Could you check a few things on this model? Use its own coordinates, in mm. A direction names the side the tool comes from. Give positions to 0.01 mm unless a question says otherwise; leave off trailing zeros. Loops run counter-clockwise (first coordinate to the right, second up) from the corner with the lowest first, then second, coordinate; pieces in that order, holes last. Notation, with made-up numbers: M 30,57.25 L 56,57.25 A34 ccw 56,90.25 Z; hole C 44.25,18 d6. An arc over 180 degrees is marked long. Use CSV: the item, a comma, the result in double quotes.
```python
from build123d import *

# Parameters (mm, degrees)
ESQUISSE1_R             = 12.5
BOSS_EXTRU_1_DEPTH      = 17
ESQUISSE2_R             = 12.5
BOSS_EXTRU_2_DEPTH      = 7
BOSS_EXTRU_2_TAPER      = 35
ESQUISSE3_R             = 1.5
ENL_V_MAT_EXTRU_1_DEPTH = 10
CONG_1_SIZE             = 0.5
ESQUISSE4_R             = 3.5
BOSS_EXTRU_3_DEPTH      = 2
ESQUISSE5_R             = 1.15
BOSS_EXTRU_4_DEPTH      = 13


with BuildPart() as part:
    # Esquisse1 → Boss.-Extru.1 (new body)
    with BuildSketch(Plane.XY):
        Circle(ESQUISSE1_R)
    extrude(amount=BOSS_EXTRU_1_DEPTH)

    # Esquisse2 → Boss.-Extru.2 (add)
    with BuildSketch(Plane.XY.offset(17)):
        Circle(ESQUISSE2_R)
    extrude(amount=BOSS_EXTRU_2_DEPTH, taper=BOSS_EXTRU_2_TAPER)

    # Esquisse3 → Enlèv. mat.-Extru.1 (cut)
    with BuildSketch(Plane(origin=(0, 0, 0), x_dir=(-1, 0, 0), z_dir=(0, 0, -1))):
        with Locations((-8, 0)):
            Circle(ESQUISSE3_R)
        with Locations((8, 0)):
            Circle(ESQUISSE3_R)
    extrude(amount=-ENL_V_MAT_EXTRU_1_DEPTH, mode=Mode.SUBTRACT)

    # Congé1
    # a fillet whose section is not a circle: 0.5 mm, written as the material it takes off along each edge
    with BuildSketch(Plane(origin=(-8, 0, 0), x_dir=(-1, 0, 0), z_dir=(0, -1, 0))) as cong_1_piece_1:
        with BuildLine():
            Bezier((1.5 + CONG_1_SIZE, 0), (1.5, 0), (1.5, -CONG_1_SIZE), weights=[1, 0.035355339, 1])
            Line((1.5, -CONG_1_SIZE), (1.5, 0))
            Line((1.5, 0), (1.5 + CONG_1_SIZE, 0))
        make_face()
    revolve(axis=Axis((-8, 0, 0), (0, 0, -1)), mode=Mode.SUBTRACT)
    with BuildSketch(Plane(origin=(8, 0, 0), x_dir=(-1, 0, 0), z_dir=(0, -1, 0))) as cong_1_piece_2:
        with BuildLine():
            Bezier((1.5 + CONG_1_SIZE, 0), (1.5, 0), (1.5, -CONG_1_SIZE), weights=[1, 0.035355339, 1])
            Line((1.5, -CONG_1_SIZE), (1.5, 0))
            Line((1.5, 0), (1.5 + CONG_1_SIZE, 0))
        make_face()
    revolve(axis=Axis((8, 0, 0), (0, 0, -1)), mode=Mode.SUBTRACT)

    # Esquisse4 → Boss.-Extru.3 (add)
    with BuildSketch(Plane(origin=(0, 0, 0), x_dir=(-1, 0, 0), z_dir=(0, 0, -1))):
        with Locations(Location((0, 0, 0), (0, 0, 180))):
            Circle(ESQUISSE4_R)
    extrude(amount=BOSS_EXTRU_3_DEPTH)

    # Esquisse5 → Boss.-Extru.4 (add)
    with BuildSketch(Plane(origin=(0, 0, -2), x_dir=(-1, 0, 0), z_dir=(0, 0, -1))):
        with Locations(Location((0, 0, 0), (0, 0, 180))):
            Circle(ESQUISSE5_R)
    extrude(amount=BOSS_EXTRU_4_DEPTH)


solid = part.part
```
1. Please list where these lines run through material, in increasing order: line 1 (Z direction, x = -3.75, y = -1.5); line 2 (Y direction, x = -8, z = 7.5); line 3 (X direction, y = -0.5, z = 11).
Outcome:
line 1,"0 to 24"
line 2,"-9.6 to -1.5, 1.5 to 9.6"
line 3,"-12.49 to 12.49"
2. I want a section at B-B, the plane z = 3. List the corners of the cut face in (x, y) for me.
Outcome:
outline,"C 0,0 d25; hole C -8,0 d3; hole C 8,0 d3"
3. I want a section at A-A, the plane x = 0. List the corners of the cut face in (y, z) for me.
Outcome:
outline,"M -12.5,0 L -3.5,0 L -3.5,-2 L -1.15,-2 L -1.15,-15 L 1.15,-15 L 1.15,-2 L 3.5,-2 L 3.5,0 L 12.5,0 L 12.5,17 L 7.6,24 L -7.6,24 L -12.5,17 Z"
4. I'm going to push flat-ended pins straight in: pin 1 Ø3.5 at (x, y) = (8.5, -0.5) entering from -Z; pin 2 Ø6 at (x, y) = (-6, -9) entering from +Z; pin 3 Ø6 at (y, z) = (-8, 18) entering from -X. Where does each tip first touch, or does it pass through?
Outcome:
pin 1,"z = 0"
pin 2,"z = 23.69"
pin 3,"x = -11.38"
5. I want a section at C-C, the plane z = -4.5. List the corners of the cut face in (x, y) for me.
Outcome:
outline,"C 0,0 d2.3"
6. Which directions (+Z, -Z, +X, -X, +Y, -Y) give clear straight access to the entire face, cutting with the end or side of a thin tool? Please do faces 4 (the face through (7.475, 2.354, 23.66)), 5 (the face through (-0.91, 0.7, -8.41)).
Outcome:
face 4,"+Z"
face 5,"-Z"
7. If we mould it in two halves opening along X, with no side actions, what happens to faces 1 (the face through (11.923, 3.755, 8.381)), 2 (the face through (8, 0, 10)), 3 (the face through (0, 0, 24))? For each: +X half, -X half, draft (parallel to the pull), parting line (faces both ways), or undercut.
Outcome:
face 1,"parting line"
face 2,"undercut"
face 3,"draft"
8. I want a section at D-D, the plane z = 16. List the corners of the cut face in (x, y) for me.
Outcome:
outline,"C 0,0 d25"
